from build123d import *

# Parameters (mm, degrees)
BOSS_EXTRUDE1_DEPTH = 6
BOSS_EXTRUDE2_DEPTH = 30
CUT_EXTRUDE1_DEPTH  = 3
CUT_EXTRUDE2_DEPTH  = 3
SKETCH6_W           = 100
SKETCH6_H           = 20
CUT_EXTRUDE3_DEPTH  = 3
SHELL4_START        = 2
SHELL4_DEPTH        = 34
CUT_EXTRUDE4_REACH  = 197.438
SKETCH7_W           = 90
SKETCH7_H           = 30
BOSS_EXTRUDE3_DEPTH = 6


# Read off the part's stored shape, not the designer's step: Shell4
with BuildPart() as part:
    # Sketch2 → Boss-Extrude1 (new body)
    with BuildSketch(Plane(origin=(0, 0, 0), x_dir=(1, 0, 0), z_dir=(0, 1, 0))):
        with BuildLine():
            Line((50, -50), (0, -50))
            Line((0, -50), (-50, -50))
            Line((-50, -50), (-50, -141.421356237))
            ThreePointArc((-50, -141.421356237), (0, -150), (50, -141.421356237))
            Line((50, -141.421356237), (50, -50))
        make_face()
        with BuildLine():
            Line((-50, -141.421356237), (-50, -50))
            Line((-50, -50), (-70, -50))
            Line((-70, -50), (-70, -132.664991614))
            ThreePointArc((-70, -132.664991614), (-60.159525267, -137.407538074), (-50, -141.421356237))
        make_face()
        with BuildLine():
            Line((70, -50), (50, -50))
            Line((50, -50), (50, -141.421356237))
            ThreePointArc((50, -141.421356237), (60.159525267, -137.407538074), (70, -132.664991614))
            Line((70, -132.664991614), (70, -50))
        make_face()
        Polygon((-50, -50), (0, -50), (50, -50), (50, -30), (-50, -30), align=None)
    extrude(amount=BOSS_EXTRUDE1_DEPTH)

    # Sketch3 → Boss-Extrude2 (add)
    with BuildSketch(Plane(origin=(0, 6, 0), x_dir=(-1, 0, 0), z_dir=(0, 1, 0))):
        with BuildLine():
            Line((50, 50), (-50, 50))
            Line((-50, 50), (-50, 141.421356237))
            ThreePointArc((-50, 141.421356237), (0, 150), (50, 141.421356237))
            Line((50, 141.421356237), (50, 50))
        make_face()
    extrude(amount=BOSS_EXTRUDE2_DEPTH)

    # Sketch4 → Cut-Extrude1 (cut)
    with BuildSketch(Plane.XZ):
        with BuildLine():
            Line((-50, 141.421356237), (-50, 50))
            Line((-50, 50), (-70, 50))
            Line((-70, 50), (-70, 132.664991614))
            ThreePointArc((-70, 132.664991614), (-60.159525267, 137.407538074), (-50, 141.421356237))
        make_face()
    extrude(amount=-CUT_EXTRUDE1_DEPTH, mode=Mode.SUBTRACT)

    # Sketch5 → Cut-Extrude2 (cut)
    with BuildSketch(Plane.XZ):
        with BuildLine():
            Line((50, 141.421356237), (50, 50))
            Line((50, 50), (70, 50))
            Line((70, 50), (70, 132.664991614))
            ThreePointArc((70, 132.664991614), (60.159525267, 137.407538074), (50, 141.421356237))
        make_face()
    extrude(amount=-CUT_EXTRUDE2_DEPTH, mode=Mode.SUBTRACT)

    # Sketch6 → Cut-Extrude3 (cut)
    with BuildSketch(Plane.XZ):
        with Locations((0, 40)):
            Rectangle(SKETCH6_W, SKETCH6_H)
    extrude(amount=-CUT_EXTRUDE3_DEPTH, mode=Mode.SUBTRACT)

    # Shell4 outline → Shell4 (cut)
    with BuildSketch(Plane(origin=(0, 0, 0), x_dir=(1, 0, 0), z_dir=(0, 1, 0)).offset(SHELL4_START)):
        with BuildLine():
            Line((-48, -52), (-48, -140))
            ThreePointArc((-48, -140), (0, -148), (48, -140))
            Line((48, -140), (48, -52))
            Line((48, -52), (-48, -52))
        make_face()
    extrude(amount=SHELL4_DEPTH, mode=Mode.SUBTRACT)

    # Sketch7 → Cut-Extrude4 (cut, up to next)
    with BuildSketch(Plane.ZY.offset(50), mode=Mode.PRIVATE) as cut_extrude4_sk1:
        with Locations((95, 21)):
            Rectangle(SKETCH7_W, SKETCH7_H)
    cut_extrude4_tool1 = extrude(cut_extrude4_sk1.sketch, amount=-CUT_EXTRUDE4_REACH, mode=Mode.PRIVATE) & part.part
    add(cut_extrude4_tool1.solids().sort_by_distance((-50, 21, 95))[0], mode=Mode.SUBTRACT)

    # Sketch8 → Boss-Extrude3 (add)
    with BuildSketch(Plane.XZ):
        with BuildLine():
            Line((-48, 140), (-48, 52))
            Line((-48, 52), (48, 52))
            Line((48, 52), (48, 140))
            ThreePointArc((48, 140), (0, 148), (-48, 140))
        make_face()
    extrude(amount=-BOSS_EXTRUDE3_DEPTH)


solid = part.part
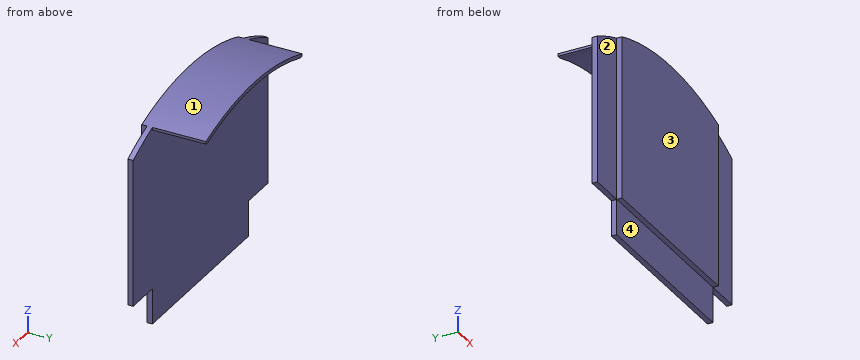
Here's how the part is built. I have some questions about the finished solid (model axes, mm). Face numbers are marked on the shaded views. A direction names the side the tool comes from. Give positions to 0.01 mm unless a question says otherwise; leave off trailing zeros. Order: outer loops, then holes, each group sorted by start corner. A loop starts at its lowest first (then second) coordinate and runs counter-clockwise, first axis right, second up. Notation, with made-up numbers: M 48,-34.5 L 75,-34.5 A17 ccw 75,-11.5 Z; hole C -23,-6 d1. An arc over 180 degrees is marked long. Answer as a JSON object with one key per item and string values. Group by question number.
1) We'd pull the mould along Y, two halves only. Please class the marked faces 1 and 2: pulls with the +Y half, pulls with the -Y half, needs draft (parallel to the pull), parting line crosses it, or undercut.
2) Suppose I cut it at C-C, the plane y = 15.5. Write out the boundary of the cut face in (x, z).
3) On a 3-axis mill with a long thin cutter (end or side, diameter ignored), from which of +Z, -Z, +X, -X, +Y, -Y can I reach the whole of each face in a straight line? I mean the marked faces 3 and 4. Say none if no direction works.
4) I'm going to push flat-ended pins straight in: pin 1 Ø16 at (x, z) = (-59, 82) entering from -Y; pin 2 Ø0.9 at (y, z) = (4, 42.5) entering from -X; pin 3 Ø3.5 at (x, y) = (-65, 4.5) entering from -Z. Where does each tip first touch, or does it pass through?
5) Suppose I cut it at B-B, the plane x = 7. Write out the boundary of the cut face in (y, z), plus the area to 3 significant figures.
6) Please list where these lines run through material, in increasing order: L1, parallel to Y at x = 59.5, z = 68.5; L2, parallel to Z at x = -1, y = 16; L3, parallel to Y at x = 31, z = 60.5. Write a range as [from, to].
7) Suppose I cut it at A-A, the plane z = 69. Write out the boundary of the cut face in (x, y).
Results found:
{
 "1": {"face 1": "needs draft", "face 2": "pulls with the -Y half"},
 "2": {"outline": "M -50,140 L -48,140 A148 cw 48,140 L 50,140 L 50,141.42 A150 ccw -50,141.42 Z"},
 "3": {"face 3": "+Z, -Z, +X, -X, -Y", "face 4": "-Z, +X, -X, -Y"},
 "4": {"pin 1": "y = 3", "pin 2": "x = -50", "pin 3": "z = 50"},
 "5": {"outline": "M 0,50 L 3,50 L 3,30 L 6,30 L 6,147.83 L 36,147.83 L 36,149.84 L 0,149.84 Z", "area": "719 mm²"},
 "6": {"L1": "[3, 6]", "L2": "[148, 150]", "L3": "[0, 6]"},
 "7": {"outline": "M -70,3 L -50,3 L -50,0 L 50,0 L 50,3 L 70,3 L 70,6 L -70,6 Z"}
}
